```python
from build123d import *

# Parameters (mm, degrees)
SKETCH1_R           = 8.6995
BOSS_EXTRUDE1_DEPTH = 5.7404
SKETCH2_R           = 6.468056998
BOSS_EXTRUDE2_DEPTH = 7.366
SKETCH3_R           = 0.508
CUT_EXTRUDE1_DEPTH  = 7.366
CIRPATTERN1_COUNT   = 20
SKETCH4_R           = 8.6995
BOSS_EXTRUDE3_DEPTH = 1.1938
SKETCH5_R           = 3.175
CUT_EXTRUDE2_DEPTH  = 15.3002


with BuildPart() as part:
    # Sketch1 → Boss-Extrude1 (new body)
    with BuildSketch(Plane.XY):
        Circle(SKETCH1_R)
    extrude(amount=BOSS_EXTRUDE1_DEPTH)

    # Sketch2 → Boss-Extrude2 (add)
    with BuildSketch(Plane.XY.offset(5.7404)):
        Circle(SKETCH2_R)
    extrude(amount=BOSS_EXTRUDE2_DEPTH)

    # Sketch3 → Cut-Extrude1 (cut)
    with BuildSketch(Plane.XY.offset(13.1064)):
        with Locations((0, 6.468056998)):
            Circle(SKETCH3_R)
    cut_extrude1 = extrude(amount=-CUT_EXTRUDE1_DEPTH, mode=Mode.SUBTRACT)

    # CirPattern1: Cut-Extrude1 ×20 about axis
    cirpattern1_axis = Axis((0, 0, 0), (0, 0, 1))
    for i in range(1, CIRPATTERN1_COUNT):
        add(cut_extrude1.rotate(cirpattern1_axis, i * 360 / CIRPATTERN1_COUNT), mode=Mode.SUBTRACT)

    # Sketch4 → Boss-Extrude3 (add)
    with BuildSketch(Plane.XY.offset(13.1064)):
        Circle(SKETCH4_R)
    extrude(amount=BOSS_EXTRUDE3_DEPTH)

    # Sketch5 → Cut-Extrude2 (cut, through all)
    with BuildSketch(Plane(origin=(0, 0, 0), x_dir=(-1, 0, 0), z_dir=(0, 0, -1))):
        Circle(SKETCH5_R)
    extrude(amount=-CUT_EXTRUDE2_DEPTH, mode=Mode.SUBTRACT)


solid = part.part
```
Verification items for the finished model (mm, model axes). A direction names the side the tool comes from. Coordinates: 2 decimals unless noted, no trailing zeros. Loops run counter-clockwise (first coordinate to the right, second up) from the corner with the lowest first, then second, coordinate; pieces in that order, holes last. Notation, with made-up numbers: (73, 53.5) - (125, 53.5) arc R17 ccw to (125, 74.5) - close; hole circle Ø10 at (9.5, 45). An arc over 180 degrees is marked (long way). Put each result on its own line as item: value.
Item 1: Draft check along Z on faces 6 (the face through (3.49, 4.83, 9.47)), 7 (the face through (3.512, -4.815, 9.475)), 8 (the face through (-1.89, -8.49, 2.83)), 9 (the face through (0, -4, 14.3)). Enter one of: pulls with the +Z half, pulls with the -Z half, needs draft (parallel to the pull), parting line crosses it, or undercut.
Conclusion:
face 6: undercut
face 7: undercut
face 8: needs draft
face 9: pulls with the +Z half
Item 2: Gauge pin test, flat ends, axial feed: pin 1 Ø1.5 at (x, z) = (3.5, 12) entering from +Y; pin 2 Ø3 at (x, z) = (-2.5, 7.5) entering from -Y; pin 3 Ø1 at (y, z) = (1.5, 2) entering from -X. Record the tip position at first contact, or that the pin passes through.
Conclusion:
pin 1: stops at y = 5.85
pin 2: stops at y = -6.39
pin 3: stops at x = -8.64
Item 3: Section check A-A (x = 0). Enter the section's corners in (y, z) (1 decimal), then the cut area to 3 significant figures.
Conclusion:
outline: (-8.7, 0) - (-3.2, 0) - (-3.2, 14.3) - (-8.7, 14.3) - (-8.7, 13.1) - (-6, 13.1) - (-6, 5.7) - (-8.7, 5.7) - close; (3.2, 0) - (8.7, 0) - (8.7, 5.7) - (6, 5.7) - (6, 13.1) - (8.7, 13.1) - (8.7, 14.3) - (3.2, 14.3) - close
area: 118 mm2
Item 4: Scan lines: line 1 along Y through (x, z) = (0, 10) (3 decimals); line 2 along Z through (x, y) = (-5, -3.5); line 3 along X through (y, z) = (2.75, 9). Record each from-to range of solid material in increasing order.
Conclusion:
line 1: y = -5.96 to -3.175, 3.175 to 5.96
line 2: z = 0 to 5.74, 13.11 to 14.3
line 3: x = -5.85 to -1.59, 1.59 to 5.85
Item 5: Set-up check for faces 1 (the face through (-5.766, -2.93, 9.372)), 2 (the face through (6.387, -1.019, 9.372)), 3 (the face through (4.83, -3.49, 9.47)), 4 (the face through (0.01, -5.96, 9.47)), 5 (the face through (-6.387, 1.019, 9.372)): record each of +Z, -Z, +X, -X, +Y, -Y from which the full face is reachable in a straight line by a thin tool's end or side.
Conclusion:
face 1: -X, -Y
face 2: +X, -Y
face 3: none
face 4: -Y
face 5: -X, +Y
